from build123d import *

# Parameters (mm, degrees)
SKETCH1_R           = 14.2875
SKETCH1_R_2         = 2.6289
BOSS_EXTRUDE1_DEPTH = 6.35
CUT_EXTRUDE4_DEPTH  = 6.35
SKETCH3_R           = 3.2639
CUT_EXTRUDE5_DEPTH  = 6.35
FILLET1_R           = 6.35
BOSS_EXTRUDE2_DEPTH = 6.35
FILLET3_R           = 6.35


with BuildPart() as part:
    # Sketch1 → Boss-Extrude1 (new body)
    with BuildSketch(Plane(origin=(0, 0, 0), x_dir=(0, 0, -1), z_dir=(1, 0, 0))):
        with BuildLine():
            Line((152.4, 0), (152.4, -50.8))
            Line((152.4, -50.8), (203.2, -50.8))
            Line((203.2, -50.8), (203.2, 0))
            ThreePointArc((203.2, 0), (200.112935412, 35.285309702), (190.945540544, 69.498493124))
            ThreePointArc((190.945540544, 69.498493124), (189.701046492, 72.826869766), (188.398540476, 76.132975421))
            Line((188.398540476, 76.132975421), (229.610721205, 92.787063794))
            ThreePointArc((229.610721205, 92.787063794), (212.273109896, 127.556455404), (189.710906338, 159.186351539))
            Line((189.710906338, 159.186351539), (155.660230842, 130.614442288))
            Line((155.660230842, 130.614442288), (116.745173131, 97.960831716))
            ThreePointArc((116.745173131, 97.960831716), (143.209155408, 52.123869843), (152.4, 0))
        make_face()
        with Locations((188.005902275, 113.300555851)):
            Circle(SKETCH1_R, mode=Mode.SUBTRACT)
        with Locations((174.895446842, 135.055462386)):
            Circle(SKETCH1_R_2, mode=Mode.SUBTRACT)
        with Locations((201.116357708, 91.545649316)):
            Circle(SKETCH1_R_2, mode=Mode.SUBTRACT)
    extrude(amount=BOSS_EXTRUDE1_DEPTH)

    # Sketch2 → Cut-Extrude4 (cut)
    with BuildSketch(Plane(origin=(6.35, 0, 0), x_dir=(0, 0, -1), z_dir=(1, 0, 0))):
        with BuildLine():
            ThreePointArc((134.46138915, 101.323924376), (129.890458655, 101.966326764), (129.248056268, 97.395396268))
            ThreePointArc((129.248056268, 97.395396268), (153.473001896, 51.351348104), (161.8361, 0))
            ThreePointArc((161.8361, 0), (165.1, -3.2639), (168.3639, 0))
            ThreePointArc((168.3639, 0), (159.663469053, 53.422649441), (134.46138915, 101.323924376))
        make_face()
        with BuildLine():
            ThreePointArc((154.746731105, 116.610025965), (150.17580061, 117.252428352), (149.533398223, 112.681497856))
            ThreePointArc((149.533398223, 112.681497856), (177.560422739, 59.410886377), (187.2361, 0))
            ThreePointArc((187.2361, 0), (190.5, -3.2639), (193.7639, 0))
            ThreePointArc((193.7639, 0), (183.750889895, 61.482187713), (154.746731105, 116.610025965))
        make_face()
    extrude(amount=-CUT_EXTRUDE4_DEPTH, mode=Mode.SUBTRACT)

    # Sketch3 → Cut-Extrude5 (cut)
    with BuildSketch(Plane(origin=(6.35, 0, 0), x_dir=(0, 0, -1), z_dir=(1, 0, 0))):
        with Locations((165.1, -38.1)):
            Circle(SKETCH3_R)
        with Locations((190.5, -38.1)):
            Circle(SKETCH3_R)
    extrude(amount=-CUT_EXTRUDE5_DEPTH, mode=Mode.SUBTRACT)

    # Fillet1
    fillet1_edges = [part.edges().sort_by_distance(p)[0] for p in [
        (3.175, 159.186351539, -189.710906338),
    ]]
    fillet(fillet1_edges, radius=FILLET1_R)

    # Sketch4 → Cut-Revolve1 (revolve, cut)
    with BuildSketch(Plane(origin=(0, 0, 0), x_dir=(1, 0, 0), z_dir=(0, 1, 0))):
        with BuildLine():
            Line((-89.242743252, 38.1), (146.392743252, 38.1))
            ThreePointArc((146.392743252, 38.1), (28.575, 155.917743252), (-89.242743252, 38.1))
        make_face()
    revolve(axis=Axis((-1000, 0, 0), (1, 0, 0)), mode=Mode.SUBTRACT)

    # Sketch5 → Boss-Extrude2 (add)
    with BuildSketch(Plane.ZY):
        with BuildLine():
            Line((-197.229722061, 79.701708643), (-229.610721205, 92.787063794))
            ThreePointArc((-229.610721205, 92.787063794), (-243.09835212, 47.262180406), (-247.65, 0))
            Line((-247.65, 0), (-203.2, -12.7))
            Line((-203.2, -12.7), (-203.2, 0))
            Line((-203.2, 0), (-212.725, 0))
            ThreePointArc((-212.725, 0), (-208.81525118, 40.597001118), (-197.229722061, 79.701708643))
        make_face()
    extrude(amount=-BOSS_EXTRUDE2_DEPTH)

    # Fillet3
    fillet3_edges = [part.edges().sort_by_distance(p)[0] for p in [
        (3.175, 0, -247.65),
    ]]
    fillet(fillet3_edges, radius=FILLET3_R)


solid = part.part
The model under review builds one solid part; all positions refer to its coordinate system, in mm. A direction names the side the tool comes from. Give positions to 0.01 mm unless a question says otherwise; leave off trailing zeros. Order: outer loops, then holes, each group sorted by start corner. A loop starts at its lowest first (then second) coordinate and runs counter-clockwise, first axis right, second up. Notation, with made-up numbers: M -3.75,57.5 L 50.25,57.5 A17 cw 50.25,64.5 Z; hole C 57.25,45 d3. An arc over 180 degrees is marked long. Answer in a Markdown table with one row per item. Add a question column.
1. For pin 1 Ø6 at (y, z) = (122.5, -156) entering from -X; pin 2 Ø1 at (x, y) = (2.5, 127.5) entering from -Z, all flat-tipped, find the tip position at first contact; note any pin that passes through.
2. Add section B-B on y = 31.5. Count the separate pieces of the cut face and the enclosed holes in it, plus the area to 3 significant figures.
3. To check wall thickness, follow line 1 along Z through (x, y) = (3.5, 67); line 2 along Z through (x, y) = (5.25, 117.5); line 3 along Z through (x, y) = (2.5, 54.5). State the ranges of each line that lie inside material, in increasing order.
4. Add section D-D on z = -235. State the section outline as (x, y) points, plus the area to 3 significant figures.
5. Machinability: for faces 1 (the flat face through (6.35, 31, -184)), 2 (the flat face through (3, -50.8, -177)), 3 (the flat face through (3, -31, -152.4)), 4 (the flat face through (3, -32, -203.2)), 5 (the cylindrical face through (3.219, 60.651, -184.027)), which of the approach directions +Z, -Z, +X, -X, +Y, -Y give a long, thin tool a straight path to every point of the face, cutting with its end or side? Answer none if there is none.
6. Mouldability with a two-part tool opening along Z and no side actions: class faces 6 (the flat face through (0, 31, -183)), 7 (the cylindrical face through (3.22, 156.51, -189.43)), 8 (the cylindrical face through (3.219, 1.05, -246.394)), 9 (the cylindrical face through (3.131, 133.456, -172.809)) as released by +Z, released by -Z, zero draft, split by the parting line, or undercut.
7. Add section A-A on z = -159. State the section outline as (x, y) points, plus the area to 3 significant figures.
The answers:
| question | item | result |
|---|---|---|
| 1 | pin 1 | x = 0 |
| 1 | pin 2 | z = -212.61 |
| 2 | separate pieces | 4 |
| 2 | enclosed holes | 0 |
| 2 | area | 463 mm2 |
| 3 | line 1 | -238.41 to -201.9, -191.84 to -181.81, -174.84 to -154.46, -147.32 to -137.79 |
| 3 | line 2 | -218 to -201.66, -174.35 to -153.72, -150.56 to -140.03 |
| 3 | line 3 | -241.58 to -205.63, -195.75 to -185.94, -179.13 to -159.3, -152.38 to -142.96 |
| 4 | outline | M 0,-3.61 L 6.35,-3.61 L 6.35,78.14 L 0,78.14 Z |
| 4 | area | 519 mm2 |
| 5 | face 1 | +Z, -Z, +X, +Y, -Y |
| 5 | face 2 | +Z, -Z, +X, -X, -Y |
| 5 | face 3 | +Z, +X, -X, -Y |
| 5 | face 4 | -Z, +X, -X, -Y |
| 5 | face 5 | +X, -X |
| 6 | face 6 | zero draft |
| 6 | face 7 | split by the parting line |
| 6 | face 8 | released by -Z |
| 6 | face 9 | undercut |
| 7 | outline | M 0,-50.8 L 6.35,-50.8 L 6.35,30.16 L 0,30.16 Z; M 0,55.37 L 6.35,55.37 L 6.35,98.88 L 0,98.88 Z; M 0,110.74 L 6.35,110.74 L 6.35,133.42 L 0,133.42 Z |
| 7 | area | 934 mm2 |
